```python
from build123d import *

# Parameters (mm, degrees)
SKETCH1_W           = 180.535384616
SKETCH1_H           = 93.243550296
SKETCH1_R           = 10.271487678
BOSS_EXTRUDE1_DEPTH = 25.4
SKETCH2_R           = 25.944815363
BOSS_EXTRUDE2_DEPTH = 19.05
SKETCH3_R           = 14.648002934
CUT_EXTRUDE1_DEPTH  = 111.894764045
FILLET2_R           = 6.35
CHAMFER1_SIZE       = 2.54


with BuildPart() as part:
    # Sketch1 → Boss-Extrude1 (new body)
    with BuildSketch(Plane(origin=(0, 0, 0), x_dir=(1, 0, 0), z_dir=(0, 1, 0))):
        Rectangle(SKETCH1_W, SKETCH1_H)
        with Locations(Location((73.073846154, 19.508402367, 0), (0, 0, 270))):
            Circle(SKETCH1_R, mode=Mode.SUBTRACT)
        with Locations(Location((-73.073846154, 19.508402367, 0), (0, 0, 270))):
            Circle(SKETCH1_R, mode=Mode.SUBTRACT)
        with Locations(Location((73.073846154, -19.508402367, 0), (0, 0, 270))):
            Circle(SKETCH1_R, mode=Mode.SUBTRACT)
        with Locations(Location((-73.073846154, -19.508402367, 0), (0, 0, 270))):
            Circle(SKETCH1_R, mode=Mode.SUBTRACT)
    extrude(amount=BOSS_EXTRUDE1_DEPTH)

    # Sketch2 → Boss-Extrude2 (add)
    with BuildSketch(Plane(origin=(0, 25.4, 0), x_dir=(1, 0, 0), z_dir=(0, 1, 0))):
        with Locations(Location((0, 0, 0), (0, 0, 90))):
            Circle(SKETCH2_R)
    extrude(amount=BOSS_EXTRUDE2_DEPTH)

    # Sketch3 → Cut-Extrude1 (cut, through all)
    with BuildSketch(Plane(origin=(0, 44.45, 0), x_dir=(1, 0, 0), z_dir=(0, 1, 0))):
        with Locations(Location((0, 0, 0), (0, 0, 270))):
            Circle(SKETCH3_R)
    extrude(amount=-CUT_EXTRUDE1_DEPTH, mode=Mode.SUBTRACT)

    # Fillet2
    fillet2_edges = [part.edges().sort_by_distance(p)[0] for p in [
        (-90.267692308, 12.7, 46.621775148),
        (-90.267692308, 12.7, -46.621775148),
        (90.267692308, 12.7, -46.621775148),
        (90.267692308, 12.7, 46.621775148),
        (0, 25.4, 25.944815363),
    ]]
    fillet(fillet2_edges, radius=FILLET2_R)

    # Chamfer1
    chamfer1_edges = [part.edges().sort_by_distance(p)[0] for p in [
        (-90.267692308, 25.4, 0),
        (0, 25.4, -46.621775148),
        (0, 25.4, 46.621775148),
        (90.267692308, 25.4, 0),
        (-88.407820368, 25.4, 44.761903208),
        (88.407820368, 25.4, 44.761903208),
        (88.407820368, 25.4, -44.761903208),
        (-88.407820368, 25.4, -44.761903208),
    ]]
    chamfer(chamfer1_edges, length=CHAMFER1_SIZE)


solid = part.part
```
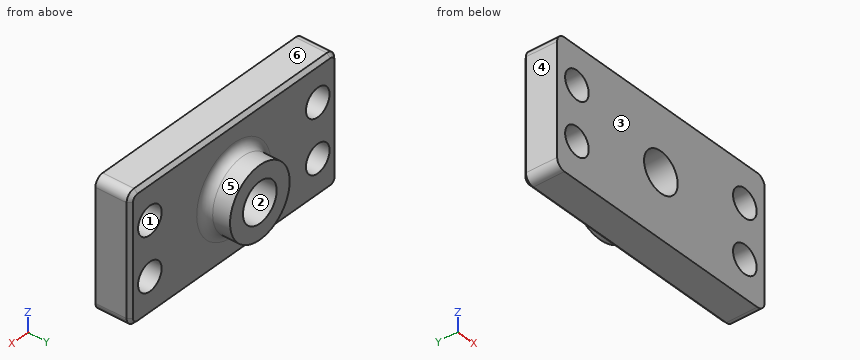
Input: part model. Units: mm. Frame: model coordinates. Face numbers are marked on the shaded views. A direction names the side the tool comes from. Round coordinates to 2 decimals unless told otherwise and drop trailing zeros. Loops run counter-clockwise (first coordinate to the right, second up) from the corner with the lowest first, then second, coordinate; pieces in that order, holes last. Notation, with made-up numbers: (54.5, -29) - (90.5, -29) arc R26 ccw to (90.5, 2) - close; hole circle Ø11 at (69, -14). An arc over 180 degrees is marked (long way). One line per item, written item: value. Start each with the question number.
(1) Contact query for flat-ended pins moving along their axis: P1, Ø6, axis at y = 35, z = 15, coming from the -X side; P2, Ø1.5, axis at x = -20, y = 24, coming from the -Z side; P3, Ø23.5, axis at x = 73.07, z = -19.51, coming from the +Y side. Output: stop coordinate, or through.
(2) Section C-C, the plane y = 38.5. Return loops of the section in (x, z).
(3) Access query for the marked faces 5 and 6. Directions: +Z, -Z, +X, -X, +Y, -Y. A direction counts if a zero-diameter tool reaches every point of the face in a straight line with its end or side. Return the directions, or none.
(4) Section B-B, the plane z = 0. Return loops of the section in (x, y), plus the area to 3 significant figures.
(5) Section A-A, the plane x = 0. Return loops of the section in (y, z).
(6) Section D-D, the plane x = -69. Return loops of the section in (y, z).
(7) Ray query, line 1 (X direction, y = 22.5, z = -19.5); line 2 (Z direction, x = -81.5, y = 16); line 3 (X direction, y = 14.5, z = 22). Return the intervals inside material, ascending. Write a range as [from, to].
(8) Draft query along X for the marked faces 1, 2, 3 and 4. Return one class per face: +X half, -X half, draft (parallel to the pull), parting line (faces both ways), or undercut.
Results below:
1. P1: x = -23
1. P2: z = -46.23
1. P3: y = 25.4
2. outline: circle Ø51.89 at (0, 0); hole circle Ø29.3 at (0, 0)
3. face 5: +Y
3. face 6: +Z, +X, -X, +Y, -Y
4. outline: (-90.27, 0) - (-14.65, 0) - (-14.65, 44.45) - (-25.94, 44.45) - (-25.94, 31.75) arc R6.35 cw to (-32.29, 25.4) - (-87.73, 25.4) - (-90.27, 22.86) - close; (14.65, 0) - (90.27, 0) - (90.27, 22.86) - (87.73, 25.4) - (32.29, 25.4) arc R6.35 cw to (25.94, 31.75) - (25.94, 44.45) - (14.65, 44.45) - close
4. area: 4,280 mm^2
5. outline: (0, -46.62) - (22.86, -46.62) - (25.4, -44.08) - (25.4, -32.29) arc R6.35 cw to (31.75, -25.94) - (44.45, -25.94) - (44.45, -14.65) - (0, -14.65) - close; (0, 14.65) - (44.45, 14.65) - (44.45, 25.94) - (31.75, 25.94) arc R6.35 cw to (25.4, 32.29) - (25.4, 44.08) - (22.86, 46.62) - (0, 46.62) - close
6. outline: (0, -46.62) - (22.86, -46.62) - (25.4, -44.08) - (25.4, -28.94) - (0, -28.94) - close; (0, -10.08) - (25.4, -10.08) - (25.4, 10.08) - (0, 10.08) - close; (0, 28.94) - (25.4, 28.94) - (25.4, 44.08) - (22.86, 46.62) - (0, 46.62) - close
7. line 1: [-90.27, -83.35], [-62.8, 62.8], [83.35, 90.27]
7. line 2: [-46.62, -25.38], [-13.63, 13.63], [25.38, 46.62]
7. line 3: [-90.27, -83.04], [-63.11, 63.11], [83.04, 90.27]
8. face 1: undercut
8. face 2: undercut
8. face 3: draft
8. face 4: -X half
